```python
from build123d import *

# Parameters (mm, degrees)
SKETCH_1_W          = 69.85
SKETCH_1_H          = 100
EXTRUDE_1_DEPTH     = 9.5
SKETCH_2_R          = 1.5
CUT_EXTRUDE_1_DEPTH = 3
SKETCH_4_R          = 1.5
CUT_EXTRUDE_3_DEPTH = 3


with BuildPart() as part:
    # 스케치1 → 보스-돌출1 (new body)
    with BuildSketch(Plane.XY):
        with Locations((34.925, 50)):
            Rectangle(SKETCH_1_W, SKETCH_1_H)
    extrude(amount=EXTRUDE_1_DEPTH)

    # 스케치2 → 컷-돌출1 (cut)
    with BuildSketch(Plane(origin=(69.85, 0, 0), x_dir=(0, 0, -1), z_dir=(1, 0, 0))):
        with Locations((-6.5, 90.6)):
            Circle(SKETCH_2_R)
        with Locations(Location((-6.5, 14, 0), (0, 0, 180))):
            Circle(SKETCH_2_R)
    cut_extrude_1 = extrude(amount=-CUT_EXTRUDE_1_DEPTH, mode=Mode.SUBTRACT)

    # 대칭 복사1: 컷-돌출1 across plane
    add(cut_extrude_1.mirror(Plane(origin=(34.925, 0, 0), x_dir=(0, 0, 1), z_dir=(1, 0, 0))), mode=Mode.SUBTRACT)

    # 스케치4 → 컷-돌출3 (cut)
    with BuildSketch(Plane.XY.offset(9.5)):
        with Locations((4.065, 90.6)):
            Circle(SKETCH_4_R)
        with Locations(Location((65.785, 90.6, 0), (0, 0, 315.234915329))):
            Circle(SKETCH_4_R)
        with Locations((4.065, 14)):
            Circle(SKETCH_4_R)
        with Locations(Location((65.785, 14, 0), (0, 0, 44.765084671))):
            Circle(SKETCH_4_R)
    extrude(amount=-CUT_EXTRUDE_3_DEPTH, mode=Mode.SUBTRACT)


solid = part.part
```
For this review, take the finished solid that the model builds, in its own axes (mm). A direction names the side the tool comes from. Round coordinates to 2 decimals unless told otherwise and drop trailing zeros. Write each loop counter-clockwise with the first axis right and the second up, starting at its lowest first coordinate (ties: lowest second). Pieces come first, ordered by that corner, then holes.
1) Take a section at A-A on y = 90.6. Give the boundary of the cut face in (x, z) (3 decimals).
Answer below:
outline: (0, 0) - (69.85, 0) - (69.85, 5) - (66.85, 5) - (66.85, 6.5) - (64.285, 6.5) - (64.285, 9.5) - (5.565, 9.5) - (5.565, 6.5) - (3, 6.5) - (3, 5) - (0, 5) - close; (0, 8) - (2.565, 8) - (2.565, 9.5) - (0, 9.5) - close; (67.285, 8) - (69.85, 8) - (69.85, 9.5) - (67.285, 9.5) - close
2) For line 1 along X through (y, z) = (90.6, 8.6) (3 decimals); line 2 along Z through (x, y) = (67.85, 90.6); line 3 along Y through (x, z) = (64.5, 6.75), list the stretches that pass through material, from the lowest coordinate up.
Answer below:
line 1: x = 0 to 2.565, 5.565 to 64.285, 67.285 to 69.85
line 2: z = 0 to 5, 8 to 9.5
line 3: y = 0 to 13.23, 14.77 to 89.83, 91.37 to 100
3) Machinability: for faces 5 (the face through (68, 14, 5)), 6 (the face through (64.3, 90.8, 8)), 7 (the face through (3, 91, 6)), which of the approach directions +Z, -Z, +X, -X, +Y, -Y give a long, thin tool a straight path to every point of the face, cutting with its end or side? Answer none if there is none.
Answer below:
face 5: +X
face 6: +Z
face 7: -X
4) Insertion check: pin 1 Ø1.3 at (y, z) = (91, 7) entering from -X; pin 2 Ø1.3 at (y, z) = (90, 6) entering from +X; pin 3 Ø1.8 at (x, y) = (65.785, 90.6) entering from +Z. Each pin has a flat end and moves straight along its axis. Give the tip position at first contact, or say it passes through.
Answer below:
pin 1: stops at x = 3
pin 2: stops at x = 66.85
pin 3: stops at z = 6.5
5) Mouldability with a two-part tool opening along Y and no side actions: class faces 1 (the face through (0, 49, 5)), 2 (the face through (66, 14, 6.5)), 3 (the face through (34, 0, 5)), 4 (the face through (66, 91, 6.5)) as +Y half, -Y half, draft (parallel to the pull), parting line (faces both ways), or undercut.
Answer below:
face 1: draft
face 2: undercut
face 3: -Y half
face 4: undercut
